```python
from build123d import *

# Parameters (mm, degrees)
SKETCH1_W                 = 31.4
SKETCH1_H                 = 20.85
SKETCH1_W_2               = 26.4
SKETCH1_H_2               = 15.85
BOSS_EXTRUDE1_DEPTH       = 4
BOSS_EXTRUDE2_START       = 4
SKETCH1_3_W               = 31.4
SKETCH1_3_H               = 20.85
SKETCH1_3_W_2             = 26.4
SKETCH1_3_H_2             = 15.85
BOSS_EXTRUDE2_DEPTH       = 13
SKETCH2_W                 = 26.4
SKETCH2_H                 = 3.2
CUT_EXTRUDE1_DEPTH        = 2.7
CUT_EXTRUDE3_DEPTH        = 47.7
F_1_0MM_DOWEL_HOLE1_D     = 3.1
F_1_0MM_DOWEL_HOLE1_DEPTH = 54.068666041
F_1_0MM_DOWEL_HOLE1_TIP   = 0.931333959


with BuildPart() as part:
    # Sketch1 → Boss-Extrude1 (new body)
    # profile 1 of 2: a face of its own
    with BuildSketch(Plane(origin=(0, 0, 0), x_dir=(1, 0, 0), z_dir=(0, 1, 0))):
        Rectangle(SKETCH1_W, SKETCH1_H)
        Rectangle(SKETCH1_W_2, SKETCH1_H_2, mode=Mode.SUBTRACT)
    # profile 2 of 2: a face of its own
    with BuildSketch(Plane(origin=(0, 0, 0), x_dir=(1, 0, 0), z_dir=(0, 1, 0))):
        Rectangle(SKETCH1_W_2, SKETCH1_H_2)
    extrude(amount=BOSS_EXTRUDE1_DEPTH)

    # Sketch1<3> → Boss-Extrude2 (add)
    with BuildSketch(Plane(origin=(0, 0, 0), x_dir=(1, 0, 0), z_dir=(0, 1, 0)).offset(BOSS_EXTRUDE2_START)):
        Rectangle(SKETCH1_3_W, SKETCH1_3_H)
        Rectangle(SKETCH1_3_W_2, SKETCH1_3_H_2, mode=Mode.SUBTRACT)
    extrude(amount=BOSS_EXTRUDE2_DEPTH)

    # Sketch2 → Cut-Extrude1 (cut)
    with BuildSketch(Plane(origin=(0, 4, 0), x_dir=(1, 0, 0), z_dir=(0, 1, 0))):
        with Locations((0, -6.325)):
            Rectangle(SKETCH2_W, SKETCH2_H)
    extrude(amount=-CUT_EXTRUDE1_DEPTH, mode=Mode.SUBTRACT)

    # Sketch3 → Cut-Extrude3 (cut)
    with BuildSketch(Plane(origin=(15.7, 0, 0), x_dir=(0, 0, -1), z_dir=(1, 0, 0))):
        Polygon((-6.804269328, 15.68296106), (-5.459911982, 15.68296106), (-7.925, 13.683572471), (-7.925, 14.773956554), align=None)
        Polygon((-3.671214098, 15.68296106), (-2.606582105, 15.68296106), (-7.925, 11.369287886), (-7.925, 12.232791762), align=None)
        Polygon((-1.037778428, 15.68296106), (0.25170719, 15.68296106), (-7.925, 8.797268756), (-7.925, 9.883158343), align=None)
        Polygon((1.375357987, 15.68296106), (2.927105978, 15.68296106), (-7.925, 6.767025954), (-7.925, 7.714901357), align=None)
        Polygon((3.956505154, 15.68296106), (5.054465963, 15.68296106), (-7.925, 4.562834301), (-7.925, 5.503509627), align=None)
        Polygon((6.716922224, 15.68296106), (7.925, 15.68296106), (7.925, 15.021555077), (-5.65165104, 4), (-6.919486669, 4), align=None)
        Polygon((7.925, 11.883512977), (-1.786125509, 4), (-3.836107122, 4), (7.925, 13.547692544), align=None)
        Polygon((1.815680904, 4), (0, 4), (7.925, 10.5), (7.925, 9.010797996), align=None)
        Polygon((4.565545231, 4), (3.069437246, 4), (7.925, 7.982480493), (7.925, 6.755388769), align=None)
    extrude(amount=-CUT_EXTRUDE3_DEPTH, mode=Mode.SUBTRACT)

    # Ø1.0mm Dowel Hole1
    with Locations(Plane(origin=(0, 4, 0), x_dir=(1, 0, 0), z_dir=(0, 1, 0))):
        with Locations((-10.35, 4.825), (10.35, 4.825)):
            Hole(F_1_0MM_DOWEL_HOLE1_D / 2, depth=F_1_0MM_DOWEL_HOLE1_DEPTH)
            with Locations((0, 0, -(F_1_0MM_DOWEL_HOLE1_DEPTH + F_1_0MM_DOWEL_HOLE1_TIP / 2))):  # 118° drill point
                Cone(0, F_1_0MM_DOWEL_HOLE1_D / 2, F_1_0MM_DOWEL_HOLE1_TIP, mode=Mode.SUBTRACT)


solid = part.part
```
Part model, mm, in its own coordinate system. A direction names the side the tool comes from. Give positions to 0.01 mm unless a question says otherwise; leave off trailing zeros. Loops run counter-clockwise (first coordinate to the right, second up) from the corner with the lowest first, then second, coordinate; pieces in that order, holes last. Notation, with made-up numbers: M 4,80.25 L 23,80.25 A31 ccw 23,114.25 Z; hole C 3,-33.75 d1. An arc over 180 degrees is marked long. Return JSON: item names as keys, results as strings.
1) Saw through at D-D, the plane x = -9.5. List the corners of the cut face in (y, z) (3 decimals), then the cut area to 3 significant figures.
Calculated:
{"outline": "M 0,-10.425 L 17,-10.425 L 17,-7.925 L 4,-7.925 L 4,-6.121 L 0,-6.121 Z; M 0,-3.529 L 4,-3.529 L 4,4.725 L 1.3,4.725 L 1.3,7.925 L 17,7.925 L 17,10.425 L 0,10.425 Z", "area": "129 mm2"}
2) 3-axis set-ups, long thin cutter, end or side, ignore diameter. For faces 1 (the face through (-13.2, 7.6, -3.4)), 2 (the face through (0, 0, 0)), 3 (the face through (14.47, 8, -3.14)): which of +Z, -Z, +X, -X, +Y, -Y reach the whole face in a straight line?
Calculated:
{"face 1": "+Y", "face 2": "+Z, -Z, +X, -X, -Y", "face 3": "+X, -X"}
3) Pull direction X, two halves, no side cores. Call faces 4 (the face through (-13.2, 11, 2)), 5 (the face through (14.47, 11.29, 2.42)): released by +X, released by -X, zero draft, split by the parting line, or undercut.
Calculated:
{"face 4": "undercut", "face 5": "zero draft"}
4) Saw through at A-A, the plane x = 10.35. List the corners of the cut face in (y, z) (3 decimals).
Calculated:
{"outline": "M 0,-10.425 L 17,-10.425 L 17,-7.925 L 4,-7.925 L 4,-6.375 L 0,-6.375 Z; M 0,-3.275 L 4,-3.275 L 4,4.725 L 1.3,4.725 L 1.3,7.925 L 17,7.925 L 17,10.425 L 0,10.425 Z"}
5) Flat gauge pins, fed straight in: pin 1 Ø1.5 at (x, z) = (-5, 0.5) entering from -Y; pin 2 Ø8 at (x, z) = (7.5, 3) entering from +Y; pin 3 Ø1 at (x, z) = (6, 6) entering from +Y. Where does each tip first touch, or does it go through?
Calculated:
{"pin 1": "stops at y = 0", "pin 2": "stops at y = 4", "pin 3": "stops at y = 1.3"}
6) Drill centre lines: line 1 (Z direction, x = 10.35, y = 3) (3 decimals); line 2 (Z direction, x = 13, y = 10) (3 decimals); line 3 (X direction, y = 11.75, z = 5.75). Where is each one in solid material? Low to high.
Calculated:
{"line 1": "z = -10.425 to -6.375, -3.275 to 4.725, 7.925 to 10.425", "line 2": "z = -10.425 to -7.925, 7.925 to 10.425", "line 3": "x = -15.7 to -13.2, 13.2 to 15.7"}
7) Saw through at C-C, the plane y = 9.5. Count the separate pieces of the cut face and the enclosed holes in it, then the cut area to 3 significant figures.
Calculated:
{"separate pieces": "12", "enclosed holes": "0", "area": "196 mm2"}
8) Saw through at B-B, the plane x = -3.5. List the corners of the cut face in (y, z) (3 decimals).
Calculated:
{"outline": "M 0,-10.425 L 17,-10.425 L 17,-7.925 L 4,-7.925 L 4,4.725 L 1.3,4.725 L 1.3,7.925 L 17,7.925 L 17,10.425 L 0,10.425 Z"}
